```python
from build123d import *

# Parameters (mm, degrees)
SKIZZE1_W                       = 20
SKIZZE1_H                       = 20
AUFSATZ_LINEAR_AUSTRAGEN1_DEPTH = 1
SKIZZE2_R                       = 3.9
SKIZZE2_R_2                     = 3.1
AUFSATZ_LINEAR_AUSTRAGEN2_DEPTH = 3
FASE1_SIZE                      = 4


with BuildPart() as part:
    # Skizze1 → Aufsatz-Linear austragen1 (new body)
    with BuildSketch(Plane(origin=(0, 0, 0), x_dir=(1, 0, 0), z_dir=(0, 1, 0))):
        Rectangle(SKIZZE1_W, SKIZZE1_H)
    extrude(amount=AUFSATZ_LINEAR_AUSTRAGEN1_DEPTH)

    # Skizze2 → Aufsatz-Linear austragen2 (add)
    with BuildSketch(Plane(origin=(0, 1, 0), x_dir=(1, 0, 0), z_dir=(0, 1, 0))):
        with Locations(Location((0, 0, 0), (0, 0, 90))):
            Circle(SKIZZE2_R)
        with Locations(Location((0, 0, 0), (0, 0, 270))):
            Circle(SKIZZE2_R_2, mode=Mode.SUBTRACT)
    extrude(amount=AUFSATZ_LINEAR_AUSTRAGEN2_DEPTH)

    # Fase1
    fase1_edges = [part.edges().sort_by_distance(p)[0] for p in [
        (10, 0.5, 10),
        (-10, 0.5, 10),
        (-10, 0.5, -10),
        (10, 0.5, -10),
    ]]
    chamfer(fase1_edges, length=FASE1_SIZE)


solid = part.part
```
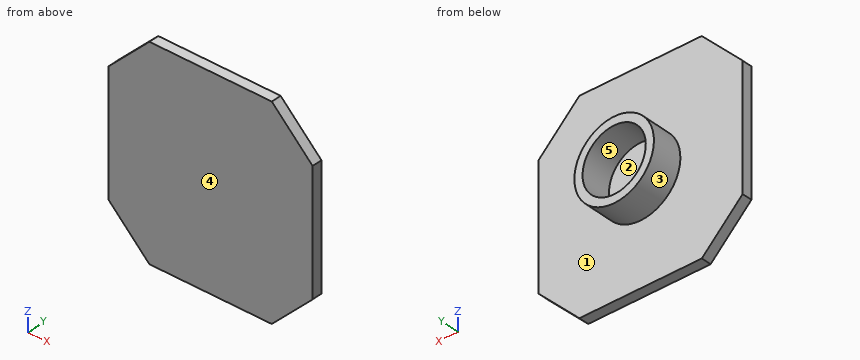
For this review, take the finished solid that the model builds, in its own axes (mm). Face numbers are marked on the shaded views. A direction names the side the tool comes from. Coordinates: 2 decimals unless noted, no trailing zeros. Order: outer loops, then holes, each group sorted by start corner. A loop starts at its lowest first (then second) coordinate and runs counter-clockwise, first axis right, second up. Notation, with made-up numbers: (46.5, 62) -> (100.5, 62) arc R19 cw to (100.5, 82) -> close; hole circle Ø7 at (-9, 3.5). An arc over 180 degrees is marked (long way). Use CSV: the item, a comma, the result in double quotes. Start each with the question number.
Item 1: Insertion check: pin 1 (8 mm diameter, centred on x = 6.5, z = -5, fed in from +Y); pin 2 (1.5 mm diameter, centred on y = 2, z = -1.5, fed in from -X). Each pin has a flat end and moves straight along its axis. Give the tip position at first contact, or say it passes through.
Item 2: Wall thickness on probe 1 along X at (y, z) = (3, 0); probe 2 along Y at (x, z) = (3.75, -5.5); probe 3 along X at (y, z) = (2.55, 1): over which ranges is each line inside the solid? List them lowest first.
Item 3: We need section D-D, the plane y = 1.65. Give the boundary of the cut face in (x, z).
Item 4: For the marked faces 4 and 5, list the 3-axis set-ups (+Z, -Z, +X, -X, +Y, -Y) from which the entire face can be reached by the end or side of a thin tool; tool diameter is ignored.
Item 5: We need section C-C, the plane z = 0. Give the boundary of the cut face in (x, y), then the cut area to 3 significant figures.
Item 6: We need section A-A, the plane x = 0. Give the boundary of the cut face in (y, z), then the cut area to 3 significant figures.
Item 7: We need section B-B, the plane y = 0.35. Give the boundary of the cut face in (x, z), then the cut area to 3 significant figures.
Item 8: Draft analysis for pull direction X (two halves, no side actions). For the marked faces 1, 2 and 3, state which applies: pulls with the +X half, pulls with the -X half, needs draft (parallel to the pull), parting line crosses it, or undercut.
Derived:
1,pin 1,"stops at y = 1"
1,pin 2,"stops at x = -3.83"
2,probe 1,"x = -3.9 to -3.1, 3.1 to 3.9"
2,probe 2,"y = 0 to 1"
2,probe 3,"x = -3.77 to -2.93, 2.93 to 3.77"
3,outline,"circle Ø7.8 at (0, 0); hole circle Ø6.2 at (0, 0)"
4,face 4,"+Z, -Z, +X, -X, -Y"
4,face 5,"+Y"
5,outline,"(-10, 0) -> (10, 0) -> (10, 1) -> (3.9, 1) -> (3.9, 4) -> (3.1, 4) -> (3.1, 1) -> (-3.1, 1) -> (-3.1, 4) -> (-3.9, 4) -> (-3.9, 1) -> (-10, 1) -> close"
5,area,"24.8 mm^2"
6,outline,"(0, -10) -> (1, -10) -> (1, -3.9) -> (4, -3.9) -> (4, -3.1) -> (1, -3.1) -> (1, 3.1) -> (4, 3.1) -> (4, 3.9) -> (1, 3.9) -> (1, 10) -> (0, 10) -> close"
6,area,"24.8 mm^2"
7,outline,"(-10, -6) -> (-6, -10) -> (6, -10) -> (10, -6) -> (10, 6) -> (6, 10) -> (-6, 10) -> (-10, 6) -> close"
7,area,"368 mm^2"
8,face 1,"needs draft"
8,face 2,"undercut"
8,face 3,"parting line crosses it"
